The listing builds one solid part. Answer for the finished solid, in the listing's coordinates (mm). Round coordinates to 2 decimals unless told otherwise and drop trailing zeros. Order: outer loops, then holes, each group sorted by start corner. A loop starts at its lowest first (then second) coordinate and runs counter-clockwise, first axis right, second up. Notation, with made-up numbers: (27.5, 74) -> (45.5, 74) arc R12 ccw to (45.5, 78) -> close; hole circle Ø1 at (26, 54.25). An arc over 180 degrees is marked (long way). Return JSON: item names as keys, results as strings. Group by question number.
(1) Each of these flat-tipped pins is pushed along its axis until it touches: pin 1 (3 mm diameter, centred on x = 17.5, z = -9, fed in from -Y); pin 2 (3 mm diameter, centred on x = -14.5, y = 2.5, fed in from -Z). Where does it stop, or does it pass through?
(2) Consider line 1 (X direction, y = 1, z = 3.5); line 2 (X direction, y = 6, z = 0); line 3 (Z direction, x = -10.5, y = 2). Determine where each line is inside the solid, lowest interval first. Write a range as [from, to].
(3) The part is cut by section A-A (x = 25.5). Determine the outline of the cut face in (y, z), plus the area to 3 significant figures.
(4) The part is cut by section C-C (x = 0). Determine the outline of the cut face in (y, z), plus the area to 3 significant figures.
(5) The part is cut by section D-D (z = 4.5). Determine the outline of the cut face in (x, y), plus the area to 3 significant figures.
(6) The part is cut by section B-B (y = 1.5). Determine the outline of the cut face in (x, z), plus the area to 3 significant figures.
(7) Determine the mould class of faces 1 (the face through (7, 4, -17.5)), 2 (the face through (-19.15, 4.06, 14.49)), 3 (the face through (27.235, 4.056, 14.272)) for opening direction X: +X half, -X half, draft (parallel to the pull), parting line (faces both ways), or undercut.
from build123d import *

# Parameters (mm, degrees)
SKETCH1_W           = 50
SKETCH1_H           = 35
SKETCH1_R           = 11.5
BOSS_EXTRUDE1_DEPTH = 8
FILLET3_R           = 10
FILLET4_R           = 2
SKETCH2_R           = 1.75
CUT_EXTRUDE1_DEPTH  = 34.974254959


with BuildPart() as part:
    # Sketch1 → Boss-Extrude1 (new body)
    with BuildSketch(Plane(origin=(0, 0, 0), x_dir=(1, 0, 0), z_dir=(0, 1, 0))):
        with Locations((3, 0)):
            Rectangle(SKETCH1_W, SKETCH1_H)
        with Locations(Location((0, 0, 0), (0, 0, 270))):
            Circle(SKETCH1_R, mode=Mode.SUBTRACT)
    extrude(amount=BOSS_EXTRUDE1_DEPTH)

    # Fillet3
    fillet3_edges = [part.edges().sort_by_distance(p)[0] for p in [
        (-22, 4, 17.5),
        (-22, 4, -17.5),
    ]]
    fillet(fillet3_edges, radius=FILLET3_R)

    # Fillet4
    fillet4_edges = [part.edges().sort_by_distance(p)[0] for p in [
        (28, 4, 17.5),
        (28, 4, -17.5),
    ]]
    fillet(fillet4_edges, radius=FILLET4_R)

    # Sketch2 → Cut-Extrude1 (cut, through all)
    with BuildSketch(Plane(origin=(0, 8, 0), x_dir=(1, 0, 0), z_dir=(0, 1, 0))):
        with Locations(Location((25.5, 4.5, 0), (0, 0, 270))):
            Circle(SKETCH2_R)
        with Locations(Location((25.5, -4.5, 0), (0, 0, 270))):
            Circle(SKETCH2_R)
        with Locations(Location((25.5, -14.5, 0), (0, 0, 270))):
            Circle(SKETCH2_R)
        with Locations(Location((25.5, 14.5, 0), (0, 0, 270))):
            Circle(SKETCH2_R)
    extrude(amount=-CUT_EXTRUDE1_DEPTH, mode=Mode.SUBTRACT)


solid = part.part
Answer below:
{
 "1": {"pin 1": "stops at y = 0", "pin 2": "stops at z = -17.45"},
 "2": {"line 1": "x = [-22, -10.95], [10.95, 24.06], [26.94, 28]", "line 2": "x = [-22, -11.5], [11.5, 28]", "line 3": "z = [-17.5, -4.69], [4.69, 17.5]"},
 "3": {"outline": "(0, -17.5) -> (8, -17.5) -> (8, -16.25) -> (0, -16.25) -> close; (0, -12.75) -> (8, -12.75) -> (8, -6.25) -> (0, -6.25) -> close; (0, -2.75) -> (8, -2.75) -> (8, 2.75) -> (0, 2.75) -> close; (0, 6.25) -> (8, 6.25) -> (8, 12.75) -> (0, 12.75) -> close; (0, 16.25) -> (8, 16.25) -> (8, 17.5) -> (0, 17.5) -> close", "area": "168 mm²"},
 "4": {"outline": "(0, -17.5) -> (8, -17.5) -> (8, -11.5) -> (0, -11.5) -> close; (0, 11.5) -> (8, 11.5) -> (8, 17.5) -> (0, 17.5) -> close", "area": "96.0 mm²"},
 "5": {"outline": "(-22, 0) -> (-10.58, 0) -> (-10.58, 8) -> (-22, 8) -> close; (10.58, 0) -> (23.75, 0) -> (23.75, 8) -> (10.58, 8) -> close; (27.25, 0) -> (28, 0) -> (28, 8) -> (27.25, 8) -> close", "area": "203 mm²"},
 "6": {"outline": "(-22, -7.5) arc R10 ccw to (-12, -17.5) -> (26, -17.5) arc R2 ccw to (28, -15.5) -> (28, 15.5) arc R2 ccw to (26, 17.5) -> (-12, 17.5) arc R10 ccw to (-22, 7.5) -> close; hole circle Ø23 at (0, 0); hole circle Ø3.5 at (25.5, -14.5); hole circle Ø3.5 at (25.5, -4.5); hole circle Ø3.5 at (25.5, 4.5); hole circle Ø3.5 at (25.5, 14.5)", "area": "1,250 mm²"},
 "7": {"face 1": "draft", "face 2": "-X half", "face 3": "undercut"}
}
